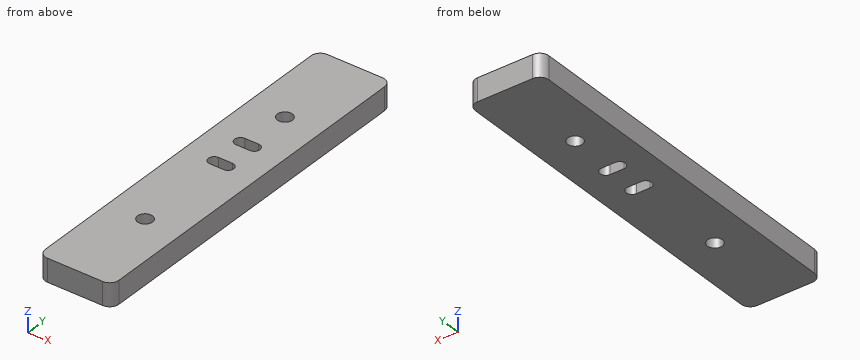
from build123d import *

# Parameters (mm, degrees)
SKETCH1_W           = 16
SKETCH1_H           = 80
SKETCH1_R           = 1.625
BOSS_EXTRUDE1_DEPTH = 5
FILLET1_R           = 2


with BuildPart() as part:
    # Sketch1 → Boss-Extrude1 (new body)
    with BuildSketch(Plane.XY):
        with Locations((8, 40)):
            Rectangle(SKETCH1_W, SKETCH1_H)
        with Locations((8, 20)):
            Circle(SKETCH1_R, mode=Mode.SUBTRACT)
        with Locations((8, 60)):
            Circle(SKETCH1_R, mode=Mode.SUBTRACT)
        with BuildLine():
            Line((6.5, 50.5), (9.5, 50.5))
            ThreePointArc((9.5, 50.5), (10.75, 49.25), (9.5, 48))
            Line((9.5, 48), (6.5, 48))
            ThreePointArc((6.5, 48), (5.25, 49.25), (6.5, 50.5))
        make_face(mode=Mode.SUBTRACT)
        with BuildLine():
            Line((6.5, 43), (9.5, 43))
            ThreePointArc((9.5, 43), (10.75, 41.75), (9.5, 40.5))
            Line((9.5, 40.5), (6.5, 40.5))
            ThreePointArc((6.5, 40.5), (5.25, 41.75), (6.5, 43))
        make_face(mode=Mode.SUBTRACT)
    extrude(amount=BOSS_EXTRUDE1_DEPTH)

    # Fillet1
    fillet1_edges = [part.edges().sort_by_distance(p)[0] for p in [
        (0, 80, 2.5),
        (16, 80, 2.5),
        (16, 0, 2.5),
        (0, 0, 2.5),
    ]]
    fillet(fillet1_edges, radius=FILLET1_R)


solid = part.part
Geometry: final body of the model. Coordinates: model frame, mm. Give positions to 0.01 mm unless a question says otherwise; leave off trailing zeros. Write each loop counter-clockwise with the first axis right and the second up, starting at its lowest first coordinate (ties: lowest second). Pieces come first, ordered by that corner, then holes. Notation, with made-up numbers: M 35.25,68 L 60.25,68 A26 ccw 60.25,89 Z; hole C -29.5,48.25 d4. An arc over 180 degrees is marked long. Answer in a Markdown table with one row per item. Add a question column.
(1) Section B-B on z = 3.95. Return loops of the section in (x, y) (3 decimals).
(2) Section C-C on y = 49.25. Return loops of the section in (x, z).
(3) Section A-A on y = 20. Return loops of the section in (x, z) (3 decimals), and give its area (4 significant figures).
(4) Ray query, line 1 (Y direction, x = 8, z = 1.1) (3 decimals); line 2 (Y direction, x = 10, z = 4); line 3 (Y direction, x = 7.25, z = 1.6). Return the intervals inside material, ascending.
Result set:
| question | item | result |
|---|---|---|
| 1 | outline | M 0,2 A2 ccw 2,0 L 14,0 A2 ccw 16,2 L 16,78 A2 ccw 14,80 L 2,80 A2 ccw 0,78 Z; hole C 8,20 d3.25; hole C 8,60 d3.25; hole M 6.5,40.5 L 9.5,40.5 A1.25 ccw 9.5,43 L 6.5,43 A1.25 ccw Z; hole M 6.5,48 L 9.5,48 A1.25 ccw 9.5,50.5 L 6.5,50.5 A1.25 ccw Z |
| 2 | outline | M 0,0 L 5.25,0 L 5.25,5 L 0,5 Z; M 10.75,0 L 16,0 L 16,5 L 10.75,5 Z |
| 3 | outline | M 0,0 L 6.375,0 L 6.375,5 L 0,5 Z; M 9.625,0 L 16,0 L 16,5 L 9.625,5 Z |
| 3 | area | 63.75 mm^2 |
| 4 | line 1 | y = 0 to 18.375, 21.625 to 40.5, 43 to 48, 50.5 to 58.375, 61.625 to 80 |
| 4 | line 2 | y = 0 to 40.6, 42.9 to 48.1, 50.4 to 80 |
| 4 | line 3 | y = 0 to 18.56, 21.44 to 40.5, 43 to 48, 50.5 to 58.56, 61.44 to 80 |
